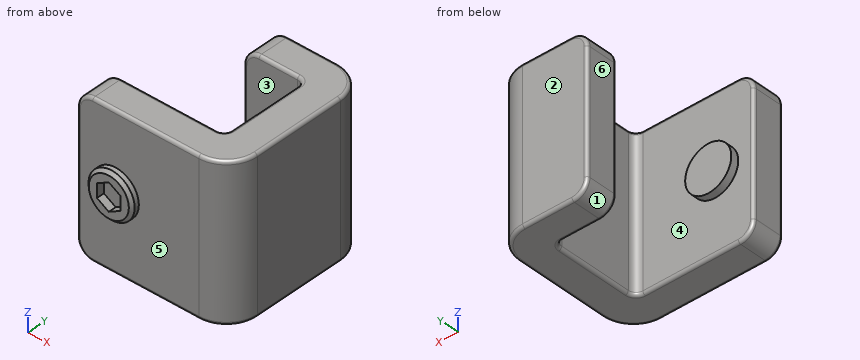
Autodesk Inventor part; units mm, degrees
ref_plane "YZ Plane" through (0, 0, 0) normal (1, 0, 0) x (0, 1, 0)
ref_plane "XZ Plane" through (0, 0, 0) normal (0, 1, 0) x (-1, 0, 0)
ref_plane "XY Plane" through (0, 0, 0) normal (0, 0, 1) x (1, 0, 0)
sketch "Эскиз1" plane through (0, 0, 0) normal (0, 0, 1) x (1, 0, 0)
  line L0 (-2, 0) -> (-9.9, 0)
  line L1 (-6.2, 10) -> (-2, 10)
  line L2 (0, 8) -> (0, 2)
  line L3 (-6.2, 7.9) -> (-2.7, 7.9)
  line L4 (-2.2, 7.4) -> (-2.2, 2.6)
  line L5 (-2.7, 2.1) -> (-9.9, 2.1)
  line L6 (0, 5) -> (-10, 5) construction
  line L7 (-6.2, 10) -> (-6.2, 7.9)
  line L8 (-9.9, 0) -> (-9.9, 2.1)
  arc A0 (0, 8) -> (-2, 10) centre (-2, 8) ccw
  arc A1 (-2, 0) -> (0, 2) centre (-2, 2) ccw
  arc A2 (-2.2, 7.4) -> (-2.7, 7.9) centre (-2.7, 7.4) ccw
  arc A3 (-2.7, 2.1) -> (-2.2, 2.6) centre (-2.7, 2.6) ccw
  point P0 (0, 0)
  dimension "d0" = 10
  dimension "d1" = 5.8
  dimension "d2" = 2.1
  dimension "d3" = 2.2
  dimension "d5" = 6.2
  dimension "d6" = 9.9
  dimension "d7" = 2
  dimension "d8" = 2.1
  dimension "d9" = 0.5
extrude "Выдавливание1" add sketch "Эскиз1" along normal mid plane 9.9
fillet "Сопряжение1" radius 1 4 edges at (-6.2, 8.95, 4.95) (-6.2, 8.95, -4.95) (-9.9, 1.05, 4.95) (-9.9, 1.05, -4.95)
fillet "Сопряжение2" radius 0.2 32 edges at (-9.6071, 2.1, 4.6571) (-9.9, 2.1, 0) (-9.6071, 2.1, -4.6571) (-5.8, 2.1, -4.95) (-2.3464, 2.2464, -4.95) (-2.2, 5, -4.95) (-2.3464, 7.7536, -4.95) (-3.95, 7.9, -4.95) (-5.9071, 7.9, -4.6571) (-6.2, 7.9, 0) (-5.9071, 7.9, 4.6571) (-3.95, 7.9, 4.95) (-2.3464, 7.7536, 4.95) (-2.2, 5, 4.95) (-2.3464, 2.2464, 4.95) (-5.8, 2.1, 4.95) (-0.5858, 0.5858, 4.95) (0, 5, 4.95) (-0.5858, 9.4142, 4.95) (-3.6, 10, 4.95) (-5.9071, 10, 4.6571) (-6.2, 10, 0) (-5.9071, 10, -4.6571) (-3.6, 10, -4.95) (-0.5858, 9.4142, -4.95) (0, 5, -4.95) (-0.5858, 0.5858, -4.95) (-5.45, 0, -4.95) (-9.6071, 0, -4.6571) (-9.9, 0, 0) (-9.6071, 0, 4.6571) (-5.45, 0, 4.95)
sketch "Эскиз2" plane through (-8.9, 0, -4.75) normal (0, -1, 0) x (1, 0, 0)
  line L0 (-1, 8.7) -> (-1, 0.8) construction
  line L1 (-1, 4.75) -> (9.4252, 4.75) construction
  circle A0 centre (1.5, 4.75) radius 1.5
  point P0 (8.9, 4.75)
  dimension "d14" = 3
  dimension "d15" = 2.5
extrude "Выдавливание2" add sketch "Эскиз2" against normal blind 2.6 and the other way blind 0.5
chamfer "Фаска1" distance 0.2 angle 45 1 edges at (-8.9, -0.5, 0)
sketch "Эскиз3" plane through (-7.4, -0.5, 0) normal (0, -1, 0) x (1, 0, 0)
  line L0 (0.004, 0.8904) -> (0.7731, 0.4417)
  line L1 (0.7731, 0.4417) -> (0.7691, -0.4487)
  line L2 (0.7691, -0.4487) -> (-0.004, -0.8904)
  line L3 (-0.004, -0.8904) -> (-0.7731, -0.4417)
  line L4 (-0.7731, -0.4417) -> (-0.7691, 0.4487)
  line L5 (-0.7691, 0.4487) -> (0.004, 0.8904)
  point P0 (7.4, 0)
  point P1 (0, 0)
extrude "Выдавливание3" cut sketch "Эскиз3" against normal blind 0.5
properties part number "скоба"
Work out the finished part from the listing and answer in its coordinate system (mm). Face numbers are marked on the shaded views. A direction names the side the tool comes from. Coordinates: 2 decimals unless noted, no trailing zeros. Order: outer loops, then holes, each group sorted by start corner. A loop starts at its lowest first (then second) coordinate and runs counter-clockwise, first axis right, second up. Notation, with made-up numbers: (86, 17) - (116, 17) arc R20 ccw to (116, 54) - close; hole circle Ø10 at (-18.5, 83.5). An arc over 180 degrees is marked (long way). Put each result on its own line as item: value. Start each with the question number.
1) Flat-ended cylindrical pins translate along their axes: pin 1 (0.9 mm diameter, centred on y = 9, z = -1.5, fed in from -X); pin 2 (2.5 mm diameter, centred on x = -8, z = 0, fed in from +Y); pin 3 (1 mm diameter, centred on x = -3.5, z = 1, fed in from -Y). Find the tip coordinate at first contact, or state that the pin passes through.
2) Find section B-B (y = 6). Give the vertices of the cut face in (x, z), plus the area to 3 significant figures.
3) Find section A-A (x = -3.75). Give the vertices of the cut face in (y, z), plus the area to 3 significant figures.
4) For the marked faces 1, 2 and 3, determine the directions among +Z, -Z, +X, -X, +Y, -Y from which every point of the face is accessible in a straight line to the end or side of a thin tool.
5) Find the intervals of material crossed by line 1 (Y direction, x = -4.25, z = -1.5); line 2 (X direction, y = 6, z = 3.25); line 3 (Y direction, x = -7.25, z = 4), in increasing order. Write a range as from..to.
6) For a pull along Y with two mould halves and no side action, classify the marked faces 4, 5 and 6 as released by +Y, released by -Y, zero draft, split by the parting line, or undercut.
Results list:
1. pin 1: stops at x = -6.2
1. pin 2: stops at y = 2.6
1. pin 3: stops at y = 0
2. outline: (-2.2, -4.75) arc R0.2 ccw to (-2, -4.95) - (-0.2, -4.95) arc R0.2 ccw to (0, -4.75) - (0, 4.75) arc R0.2 ccw to (-0.2, 4.95) - (-2, 4.95) arc R0.2 ccw to (-2.2, 4.75) - close
2. area: 21.7 mm^2
3. outline: (0, -4.75) arc R0.2 ccw to (0.2, -4.95) - (1.9, -4.95) arc R0.2 ccw to (2.1, -4.75) - (2.1, 4.75) arc R0.2 ccw to (1.9, 4.95) - (0.2, 4.95) arc R0.2 ccw to (0, 4.75) - close; (7.9, -4.75) arc R0.2 ccw to (8.1, -4.95) - (9.8, -4.95) arc R0.2 ccw to (10, -4.75) - (10, 4.75) arc R0.2 ccw to (9.8, 4.95) - (8.1, 4.95) arc R0.2 ccw to (7.9, 4.75) - close
3. area: 41.5 mm^2
4. face 1: -Z, -X, +Y
4. face 2: +Z, -Z, +X, -X, +Y
4. face 3: +Z, -Z, -X
5. line 1: y = 0..2.1, 7.9..10
5. line 2: x = -2.2..0
5. line 3: y = 0..2.1
6. face 4: undercut
6. face 5: released by -Y
6. face 6: zero draft
